Source: CAD feature listing. Evaluate the final solid. Frame: model axes, mm. A direction names the side the tool comes from. Round coordinates to 2 decimals unless told otherwise and drop trailing zeros. Loops run counter-clockwise (first coordinate to the right, second up) from the corner with the lowest first, then second, coordinate; pieces in that order, holes last. Notation, with made-up numbers: M 54,86.25 L 79,86.25 A31 cw 79,119.25 Z; hole C 28,23 d8. An arc over 180 degrees is marked long. Answer as a JSON object with one key per item and string values.
from build123d import *

# Parameters (mm, degrees)
SKETCH1_W           = 60
SKETCH1_H           = 60
SKETCH1_R           = 28.75
SKETCH1_R_2         = 2.1
BOSS_EXTRUDE4_DEPTH = 14
SKETCH1_8_R         = 28.75
BOSS_EXTRUDE5_DEPTH = 2
CUT_EXTRUDE2_START  = -2
CUT_EXTRUDE2_DEPTH  = 2


with BuildPart() as part:
    # Sketch1 → Boss-Extrude4 (new body)
    with BuildSketch(Plane(origin=(0, 0, 0), x_dir=(1, 0, 0), z_dir=(0, 1, 0))):
        Rectangle(SKETCH1_W, SKETCH1_H)
        with Locations(Location((0, 0, 0), (0, 0, 270))):
            Circle(SKETCH1_R, mode=Mode.SUBTRACT)
        with Locations(Location((-25.880108191, 25.880108191, 0), (0, 0, 270))):
            Circle(SKETCH1_R_2, mode=Mode.SUBTRACT)
        with Locations(Location((-26.120769668, -25.637187677, 0), (0, 0, 270))):
            Circle(SKETCH1_R_2, mode=Mode.SUBTRACT)
        with Locations(Location((25.96435834, -25.795582877, 0), (0, 0, 270))):
            Circle(SKETCH1_R_2, mode=Mode.SUBTRACT)
        with Locations(Location((25.713774072, 26.04538007, 0), (0, 0, 270))):
            Circle(SKETCH1_R_2, mode=Mode.SUBTRACT)
    extrude(amount=BOSS_EXTRUDE4_DEPTH)

    # Sketch1_8 → Boss-Extrude5 (add)
    with BuildSketch(Plane(origin=(0, 0, 0), x_dir=(1, 0, 0), z_dir=(0, 1, 0))):
        with Locations(Location((0, 0, 0), (0, 0, 270))):
            Circle(SKETCH1_8_R)
    extrude(amount=BOSS_EXTRUDE5_DEPTH)

    # Sketch5 → Cut-Extrude2 (cut)
    with BuildSketch(Plane(origin=(0, 14, 0), x_dir=(1, 0, 0), z_dir=(0, 1, 0)).offset(CUT_EXTRUDE2_START)):
        with BuildLine():
            Line((12.5, 30), (-12.5, 30))
            Line((-12.5, 30), (-12.5, 25.890393972))
            ThreePointArc((-12.5, 25.890393972), (0, 28.75), (12.5, 25.890393972))
            Line((12.5, 25.890393972), (12.5, 30))
        make_face()
        with BuildLine():
            ThreePointArc((-25.890393972, -12.5), (-28.75, 0), (-25.890393972, 12.5))
            Line((-25.890393972, 12.5), (-30, 12.5))
            Line((-30, 12.5), (-30, -12.5))
            Line((-30, -12.5), (-25.890393972, -12.5))
        make_face()
        with BuildLine():
            Line((30, 12.5), (25.890393972, 12.5))
            ThreePointArc((25.890393972, 12.5), (28.75, 0), (25.890393972, -12.5))
            Line((25.890393972, -12.5), (30, -12.5))
            Line((30, -12.5), (30, 12.5))
        make_face()
        with BuildLine():
            ThreePointArc((12.5, -25.890393972), (0, -28.75), (-12.5, -25.890393972))
            Line((-12.5, -25.890393972), (-12.5, -30))
            Line((-12.5, -30), (12.5, -30))
            Line((12.5, -30), (12.5, -25.890393972))
        make_face()
    extrude(amount=CUT_EXTRUDE2_DEPTH, mode=Mode.SUBTRACT)


solid = part.part
Item 1: Line query: probe 1 along Y at (x, z) = (14.5, -19.5); probe 2 along Z at (x, y) = (-20.5, 8); probe 3 along Z at (x, y) = (-10, 4.5). Output: solid intervals per line, ascending. Write a range as from..to.
Answer sheet:
{"probe 1": "y = 0..2", "probe 2": "z = -30..-20.16, 20.16..30", "probe 3": "z = -30..-26.95, 26.95..30"}
Item 2: Section B-B on y = 8.75. Return the cut outline in (x, z), then the cut area to 3 significant figures.
Answer sheet:
{"outline": "M -30,-30 L 30,-30 L 30,30 L -30,30 Z; hole C 0,0 d57.5; hole C -26.12,25.64 d4.2; hole C -25.88,-25.88 d4.2; hole C 25.71,-26.05 d4.2; hole C 25.96,25.8 d4.2", "area": "948 mm²"}
Item 3: Access query for faces 4 (the flat face through (-28, 13, -12.5)), 5 (the flat face through (12.5, 13, 28)), 6 (the cylindrical face through (1.264, 7.916, -28.722)). Directions: +Z, -Z, +X, -X, +Y, -Y. A direction counts if a zero-diameter tool reaches every point of the face in a straight line with its end or side. Return the directions, or none.
Answer sheet:
{"face 4": "+X, -X, +Y", "face 5": "+Z, -Z, +Y", "face 6": "+Y"}
Item 4: Pull-direction query (X, two-part tool) for faces 1 (the flat face through (-30, 7, 0)), 2 (the flat face through (-12.5, 13, 28)), 3 (the flat face through (23, 14, 23)); classes: pulls with the +X half, pulls with the -X half, needs draft (parallel to the pull), parting line crosses it, or undercut.
Answer sheet:
{"face 1": "pulls with the -X half", "face 2": "undercut", "face 3": "needs draft"}
Item 5: Section C-C on z = 0. Return the cut outline in (x, y), then the cut area to 3 significant figures.
Answer sheet:
{"outline": "M -30,0 L 30,0 L 30,12 L 28.75,12 L 28.75,2 L -28.75,2 L -28.75,12 L -30,12 Z", "area": "145 mm²"}
Item 6: Contact query for flat-ended pins moving along their axis: pin 1 Ø3.5 at (x, z) = (25.96, 25.8) entering from -Y; pin 2 Ø4.5 at (x, z) = (28, 1) entering from +Y; pin 3 Ø12 at (x, z) = (-6, -18.5) entering from +Y. Output: stop coordinate, or through.
Answer sheet:
{"pin 1": "passes through", "pin 2": "stops at y = 12", "pin 3": "stops at y = 2"}
Item 7: Section A-A on x = 0. Return the cut outline in (y, z), then the cut area to 3 significant figures.
Answer sheet:
{"outline": "M 0,-30 L 12,-30 L 12,-28.75 L 2,-28.75 L 2,28.75 L 12,28.75 L 12,30 L 0,30 Z", "area": "145 mm²"}
